Read the model definition and answer for the solid it produces. Units are mm, in the model's axes. A direction names the side the tool comes from. Coordinates: 2 decimals unless noted, no trailing zeros. Loops run counter-clockwise (first coordinate to the right, second up) from the corner with the lowest first, then second, coordinate; pieces in that order, holes last. Notation, with made-up numbers: (52.5, 76.25) -> (89.5, 76.25) arc R11 ccw to (89.5, 92.25) -> close; hole circle Ø4 at (5.5, -28). An arc over 180 degrees is marked (long way). Answer as a JSON object with one key per item and string values. Group by question number.
Q1. Determine the mould class of faces 1 (the flat face through (3, 11.5, -6)), 2 (the cylindrical face through (0.33, 10.486, -7.493)), 3 (the cylindrical face through (2.414, 10.444, -2.451)) for opening direction X: released by +X, released by -X, zero draft, split by the parting line, or undercut.
Q2. The part is cut by section A-A on y = 14. Write down the section's boundary in (x, z) (1 decimal).
Q3. For faces 4 (the cylindrical face through (-2.6, 10.44, 1.87)), 5 (the cylindrical face through (1.802, 4.684, 5.723)), determine the directions among +Z, -Z, +X, -X, +Y, -Y from which every point of the face is accessible in a straight line to the end or side of a thin tool.
Q4. The part is cut by section D-D on y = 4.25. Write down the section's boundary in (x, z).
Q5. The part is cut by section B-B on z = 0. Write down the section's boundary in (x, y), and give its area (3 significant figures).
Q6. Straight lines are drawn through the part: line 1 along Z through (x, y) = (2, -4.15) (3 decimals); line 2 along X through (y, z) = (12, -2); line 3 along X through (y, z) = (-0.75, -2) (3 decimals). For each, find the intervals that lie inside material, in ascending order. Write a range as [from, to].
Q7. Each of these flat-tipped pins is pushed along its axis until it touches: P1, Ø1.3, axis at x = 1.5, z = -2, coming from the +Y side; P2, Ø3, axis at x = 5.5, y = 12.5, coming from the +Z side; P3, Ø4, axis at y = 3, z = 2.5, coming from the -X side. Where does it stop, or does it pass through?
Q8. The part is cut by section C-C on x = 0. Write down the section's boundary in (y, z).
from build123d import *

# Parameters (mm, degrees)
SKETCH_1_R          = 6
EXTRUDE_1_DEPTH     = 9.5
SKETCH_2_R          = 7.5
EXTRUDE_2_DEPTH     = 2
SKETCH_3_R          = 6.5
EXTRUDE_3_DEPTH     = 5
SKETCH_4_R          = 4.5
CUT_EXTRUDE_1_DEPTH = 10
EXTRUDE_START       = 10
EXTRUDE_4_DEPTH     = 10
SKETCH_6_R          = 0.6125
EXTRUDE_5_DEPTH     = 8
SKETCH_7_R          = 0.625
EXTRUDE_6_DEPTH     = 5
SKETCH_8_R          = 0.25
CUT_EXTRUDE_2_DEPTH = 3
CUT_EXTRUDE_3_DEPTH = 10


with BuildPart() as part:
    # Эскиз1 → Бобышка-Вытянуть1 (new body)
    with BuildSketch(Plane(origin=(0, 0, 0), x_dir=(1, 0, 0), z_dir=(0, 1, 0))):
        with Locations(Location((0, 0, 0), (0, 0, 270))):
            Circle(SKETCH_1_R)
    extrude(amount=EXTRUDE_1_DEPTH)

    # Эскиз2 → Бобышка-Вытянуть2 (add)
    with BuildSketch(Plane(origin=(0, 9.5, 0), x_dir=(1, 0, 0), z_dir=(0, 1, 0))):
        with Locations(Location((0, 0, 0), (0, 0, 270))):
            Circle(SKETCH_2_R)
    extrude(amount=EXTRUDE_2_DEPTH)

    # Эскиз3 → Бобышка-Вытянуть3 (add)
    with BuildSketch(Plane(origin=(0, 11.5, 0), x_dir=(1, 0, 0), z_dir=(0, 1, 0))):
        with Locations(Location((0, 0, 0), (0, 0, 270))):
            Circle(SKETCH_3_R)
    extrude(amount=EXTRUDE_3_DEPTH)

    # Эскиз4 → Вырез-Вытянуть1 (cut)
    with BuildSketch(Plane(origin=(0, 16.5, 0), x_dir=(1, 0, 0), z_dir=(0, 1, 0))):
        with Locations(Location((0, 0, 0), (0, 0, 270))):
            Circle(SKETCH_4_R)
    extrude(amount=-CUT_EXTRUDE_1_DEPTH, mode=Mode.SUBTRACT)

    # Эскиз5 → Бобышка-Вытянуть4 (add)
    with BuildSketch(Plane(origin=(0, 6.5, 0), x_dir=(1, 0, 0), z_dir=(0, 1, 0)).offset(EXTRUDE_START)):
        with BuildLine():
            ThreePointArc((-0.499227799, -4.472222222), (0, -4.5), (0.499227799, -4.472222222))
            ThreePointArc((0.499227799, -4.472222222), (0, -4), (-0.499227799, -4.472222222))
        make_face()
    extrude(amount=-EXTRUDE_4_DEPTH)

    # Эскиз6 → Бобышка-Вытянуть5 (add)
    with BuildSketch(Plane(origin=(0, 6.5, 0), x_dir=(1, 0, 0), z_dir=(0, 1, 0))):
        with Locations(Location((-2, 2, 0), (0, 0, 270))):
            Circle(SKETCH_6_R)
        with Locations(Location((-2, -2, 0), (0, 0, 270))):
            Circle(SKETCH_6_R)
        with Locations(Location((2, -2, 0), (0, 0, 270))):
            Circle(SKETCH_6_R)
        with Locations(Location((2, 2, 0), (0, 0, 270))):
            Circle(SKETCH_6_R)
    extrude(amount=EXTRUDE_5_DEPTH)

    # Эскиз7 → Бобышка-Вытянуть6 (add)
    with BuildSketch(Plane.XZ):
        with Locations(Location((2, -2, 0), (0, 0, 90))):
            Circle(SKETCH_7_R)
        with Locations(Location((-2, -2, 0), (0, 0, 90))):
            Circle(SKETCH_7_R)
        with Locations(Location((-2, 2, 0), (0, 0, 90))):
            Circle(SKETCH_7_R)
        with Locations(Location((2, 2, 0), (0, 0, 90))):
            Circle(SKETCH_7_R)
    extrude(amount=EXTRUDE_6_DEPTH)

    # Эскиз8 → Вырез-Вытянуть2 (cut)
    with BuildSketch(Plane.XZ.offset(5)):
        with Locations(Location((2, -2, 0), (0, 0, 270))):
            Circle(SKETCH_8_R)
        with Locations(Location((-2, -2, 0), (0, 0, 270))):
            Circle(SKETCH_8_R)
        with Locations(Location((-2, 2, 0), (0, 0, 270))):
            Circle(SKETCH_8_R)
        with Locations(Location((2, 2, 0), (0, 0, 270))):
            Circle(SKETCH_8_R)
    extrude(amount=-CUT_EXTRUDE_2_DEPTH, mode=Mode.SUBTRACT)

    # Эскиз9 → Вырез-Вытянуть3 (cut, symmetric)
    with BuildSketch(Plane(origin=(0, 0, 0), x_dir=(0, 0, -1), z_dir=(1, 0, 0))):
        with BuildLine():
            Line((2, -5), (2.625, -5))
            Line((2.625, -5), (2.625, -2))
            ThreePointArc((2.625, -2), (2.169101887, -2.410376179), (2, -3))
            Line((2, -3), (2, -5))
        make_face()
        with BuildLine():
            Line((-2, -5), (-2.625, -5))
            Line((-2.625, -5), (-2.625, -2))
            ThreePointArc((-2.625, -2), (-2.169101887, -2.410376179), (-2, -3))
            Line((-2, -3), (-2, -5))
        make_face()
    extrude(amount=CUT_EXTRUDE_3_DEPTH, both=True, mode=Mode.SUBTRACT)


solid = part.part
Final values:
{
 "1": {"face 1": "zero draft", "face 2": "split by the parting line", "face 3": "undercut"},
 "2": {"outline": "circle Ø13 at (0, 0); circle Ø1.2 at (-2, -2); circle Ø1.2 at (-2, 2); circle Ø1.2 at (2, -2); circle Ø1.2 at (2, 2); hole (-0.5, 4.5) arc R4.5 ccw (long way) to (0.5, 4.5) arc R0.5 cw to start"},
 "3": {"face 4": "+Y", "face 5": "-Y"},
 "4": {"outline": "circle Ø12 at (0, 0)"},
 "5": {"outline": "(-7.5, 9.5) -> (-6, 9.5) -> (-6, 0) -> (6, 0) -> (6, 9.5) -> (7.5, 9.5) -> (7.5, 11.5) -> (6.5, 11.5) -> (6.5, 16.5) -> (4.5, 16.5) -> (4.5, 6.5) -> (-4.5, 6.5) -> (-4.5, 16.5) -> (-6.5, 16.5) -> (-6.5, 11.5) -> (-7.5, 11.5) -> close", "area": "119 mm2"},
 "6": {"line 1": "z = [-1.75, -1.375], [1.375, 1.75]", "line 2": "x = [-6.18, -4.03], [-2.61, -1.39], [1.39, 2.61], [4.03, 6.18]", "line 3": "x = [-2.625, -1.375], [1.375, 2.625]"},
 "7": {"P1": "stops at y = 14.5", "P2": "stops at z = 6.09", "P3": "stops at x = -5.98"},
 "8": {"outline": "(0, -6) -> (9.5, -6) -> (9.5, -7.5) -> (11.5, -7.5) -> (11.5, -6.5) -> (16.5, -6.5) -> (16.5, -4.5) -> (6.5, -4.5) -> (6.5, 4) -> (16.5, 4) -> (16.5, 6.5) -> (11.5, 6.5) -> (11.5, 7.5) -> (9.5, 7.5) -> (9.5, 6) -> (0, 6) -> close"}
}
